Build history of the part. All positions in model axes, mm. A direction names the side the tool comes from. Give positions to 0.01 mm unless a question says otherwise; leave off trailing zeros. Order: outer loops, then holes, each group sorted by start corner. A loop starts at its lowest first (then second) coordinate and runs counter-clockwise, first axis right, second up. Notation, with made-up numbers: M -17.75,7.25 L 23.25,7.25 A15 cw 23.25,15.25 Z; hole C 50.25,46 d8. An arc over 180 degrees is marked long. Answer as CSV lines item,"result".
from build123d import *

# Parameters (mm, degrees)
BOSS_EXTRUDE1_DEPTH = 2.5
BOSS_EXTRUDE5_DEPTH = 1.25
SKETCH6_R           = 1.25
BOSS_EXTRUDE6_DEPTH = 2.5
SKETCH7_R           = 1.25
BOSS_EXTRUDE7_DEPTH = 2.5
SKETCH8_R           = 1.25
CUT_EXTRUDE3_DEPTH  = 2.5


with BuildPart() as part:
    # Sketch1 → Boss-Extrude1 (new body)
    with BuildSketch(Plane(origin=(0, 0, 0), x_dir=(1, 0, 0), z_dir=(0, 1, 0))):
        with BuildLine():
            ThreePointArc((4, 32), (0, 36), (-4, 32))
            ThreePointArc((-4, 32), (0, 28), (4, 32))
        make_face()
    extrude(amount=BOSS_EXTRUDE1_DEPTH)

    # Sketch1<4> → Boss-Extrude5 (add)
    with BuildSketch(Plane(origin=(0, 0, 0), x_dir=(1, 0, 0), z_dir=(0, 1, 0))):
        with BuildLine():
            Line((-4, 32), (-4, 0))
            ThreePointArc((-4, 0), (0, -4), (4, 0))
            Line((4, 0), (4, 32))
            ThreePointArc((4, 32), (0, 28), (-4, 32))
        make_face()
    extrude(amount=BOSS_EXTRUDE5_DEPTH)

    # Sketch6 → Boss-Extrude6 (add)
    with BuildSketch(Plane(origin=(0, 2.5, 0), x_dir=(1, 0, 0), z_dir=(0, 1, 0))):
        with Locations((0, 32)):
            Circle(SKETCH6_R)
    extrude(amount=BOSS_EXTRUDE6_DEPTH)

    # Sketch7 → Boss-Extrude7 (add)
    with BuildSketch(Plane.XZ):
        Circle(SKETCH7_R)
    extrude(amount=BOSS_EXTRUDE7_DEPTH)

    # Sketch8 → Cut-Extrude3 (cut)
    with BuildSketch(Plane(origin=(0, 1.25, 0), x_dir=(1, 0, 0), z_dir=(0, 1, 0))):
        with Locations((0, 14)):
            Circle(SKETCH8_R)
    extrude(amount=-CUT_EXTRUDE3_DEPTH, mode=Mode.SUBTRACT)


solid = part.part
Item 1: Band-saw the part on D-D (z = -21). Give the cut face in (x, y), and give its area (3 significant figures).
Geometry says:
outline,"M -4,0 L 4,0 L 4,1.25 L -4,1.25 Z"
area,"10.0 mm2"
Item 2: Drop flat-ended pins along their axis: pin 1 (2.5 mm diameter, centred on x = -0.5, z = -9, fed in from +Y); pin 2 (1.5 mm diameter, centred on x = 0, z = -14, fed in from +Y); pin 3 (4 mm diameter, centred on x = -1.5, y = -1.5, fed in from +Z); pin 4 (3 mm diameter, centred on x = -2.5, z = -23, fed in from -Y). Give the stop position or say it passes through.
Geometry says:
pin 1,"stops at y = 1.25"
pin 2,"passes through"
pin 3,"stops at z = 4"
pin 4,"stops at y = 0"
Item 3: 3-axis set-ups, long thin cutter, end or side, ignore diameter. For faces 5 (the flat face through (-4, 1, -16)), 6 (the cylindrical face through (-0.27, -1.23, -1.22)), 7 (the flat face through (1, 2.5, -33)): which of +Z, -Z, +X, -X, +Y, -Y reach the whole face in a straight line?
Geometry says:
face 5,"+Z, -Z, -X, +Y, -Y"
face 6,"-Y"
face 7,"+Y"
Item 4: Band-saw the part on B-B (x = 0). Give the cut face in (y, z), and give its area (3 significant figures).
Geometry says:
outline,"M -2.5,-1.25 L 0,-1.25 L 0,-12.75 L 1.25,-12.75 L 1.25,4 L 0,4 L 0,1.25 L -2.5,1.25 Z; M 0,-36 L 2.5,-36 L 2.5,-33.25 L 5,-33.25 L 5,-30.75 L 2.5,-30.75 L 2.5,-28 L 1.25,-28 L 1.25,-15.25 L 0,-15.25 Z"
area,"69.4 mm2"
Item 5: Band-saw the part on A-A (z = -14). Give the cut face in (x, y).
Geometry says:
outline,"M -4,0 L -1.25,0 L -1.25,1.25 L -4,1.25 Z; M 1.25,0 L 4,0 L 4,1.25 L 1.25,1.25 Z"
Item 6: Pull direction Z, two halves, no side cores. Call faces 1 (the cylindrical face through (-0.16, 0.63, -15.24)), 2 (the cylindrical face through (-1.846, 1.51, -35.549)), 3 (the cylindrical face through (0, 1, 4)), 4 (the flat face through (0, 0, -16)): released by +Z, released by -Z, zero draft, split by the parting line, or undercut.
Geometry says:
face 1,"undercut"
face 2,"split by the parting line"
face 3,"released by +Z"
face 4,"zero draft"
Item 7: Band-saw the part on C-C (y = 0.5). Give the cut face in (x, z), and give its area (3 significant figures).
Geometry says:
outline,"M -4,-32 A4 ccw 4,-32 L 4,0 A4 ccw -4,0 Z; hole C 0,-14 d2.5"
area,"301 mm2"
Item 8: Probe line 1 along X through (y, z) = (0.35, -14); line 2 along Z through (x, y) = (0, 0.3); line 3 along Y through (x, z) = (-0.75, -32). List the from-to ranges inside material, lowest first. Write a range as from..to.
Geometry says:
line 1,"x = -4..-1.25, 1.25..4"
line 2,"z = -36..-15.25, -12.75..4"
line 3,"y = 0..5"
